Read the model definition and answer for the solid it produces. Units are mm, in the model's axes. A direction names the side the tool comes from. Coordinates: 2 decimals unless noted, no trailing zeros. Loops run counter-clockwise (first coordinate to the right, second up) from the corner with the lowest first, then second, coordinate; pieces in that order, holes last.
from build123d import *

# Parameters (mm, degrees)
SKETCH021_W       = 18.9
SKETCH021_H       = 58
EXTRUDE021_DEPTH  = 10
SKETCH020_W       = 90
SKETCH020_H       = 50
EXTRUDE020_DEPTH  = 200
CYLINDER_R        = 2.5
CYLINDER_DEPTH    = 70
CYLINDER002_R     = 2.5
CYLINDER002_DEPTH = 70
BOX001_W          = 82
BOX001_H          = 58
BOX001_DEPTH      = 44.4
BOX011_W          = 5
BOX011_H          = 5
BOX011_DEPTH      = 44.4
SKETCH001_R       = 5
EXTRUDE001_DEPTH  = 4
EXTRUDE002_DEPTH  = 15
SKETCH010_R       = 12.3
EXTRUDE010_DEPTH  = 5
BOX_W             = 75.7
BOX_H             = 45
BOX_DEPTH         = 44.4
BOX008_W          = 68.15
BOX008_H          = 15
BOX008_DEPTH      = 50
BOX009_W          = 68.15
BOX009_H          = 15
BOX009_DEPTH      = 50
BOX012_W          = 30
BOX012_H          = 100
BOX012_DEPTH      = 70
EXTRUDE003_DEPTH  = 25
BOX010_W          = 40
BOX010_H          = 120
BOX010_DEPTH      = 60
TUBE_R            = 45
TUBE_R_2          = 19.07
TUBE_DEPTH        = 50
BOX002_W          = 175
BOX002_H          = 90
BOX002_DEPTH      = 50
SKETCH016_W       = 10
SKETCH016_H       = 33.333334
EXTRUDE016_DEPTH  = 80
SKETCH_W          = 20
SKETCH_H          = 100
EXTRUDE_DEPTH     = 100
BOX017_W          = 120
BOX017_H          = 100
BOX017_DEPTH      = 70


with BuildPart() as extrude021:
    # Sketch021 (on Face14 of Cut017) → Extrude021 (new body)
    with BuildSketch(Plane(origin=(0, 0, 44.4), x_dir=(1, 0, 0), z_dir=(0, 0, -1))):
        with Locations((-72.55, -19.37)):
            Rectangle(SKETCH021_W, SKETCH021_H)
    extrude(amount=-EXTRUDE021_DEPTH)


with BuildPart() as extrude020:
    # Sketch020 (on Face26 of Cut016) → Extrude020 (new body)
    with BuildSketch(Plane.YZ.offset(-92)):
        with Locations((19, 15)):
            Rectangle(SKETCH020_W, SKETCH020_H)
    extrude(amount=EXTRUDE020_DEPTH)


with BuildPart() as throughholecylinder2:
    # Cylinder → Cylinder (new body)
    with BuildSketch(Plane(origin=(-86, -18, -20), x_dir=(1, 0, 0), z_dir=(0, 0, 1))):
        Circle(CYLINDER_R)
    extrude(amount=CYLINDER_DEPTH)


with BuildPart() as throughholecylinder1:
    # Cylinder002 → Cylinder002 (new body)
    with BuildSketch(Plane(origin=(-86, 56, -20), x_dir=(1, 0, 0), z_dir=(0, 0, 1))):
        Circle(CYLINDER002_R)
    extrude(amount=CYLINDER002_DEPTH)


with BuildPart() as motorhead:
    # Box001 → Box001 (new body)
    with BuildSketch(Plane(origin=(-82, -9.63, 0), x_dir=(1, 0, 0), z_dir=(0, 0, 1))):
        with Locations((41, 29)):
            Rectangle(BOX001_W, BOX001_H)
    extrude(amount=BOX001_DEPTH)


with BuildPart() as obj1:
    # Box011 → Box011 (new body)
    with BuildSketch(Plane(origin=(75.7, 16.87, 0), x_dir=(1, 0, 0), z_dir=(0, 0, 1))):
        with Locations((2.5, 2.5)):
            Rectangle(BOX011_W, BOX011_H)
    extrude(amount=BOX011_DEPTH)


with BuildPart() as obj2:
    # Sketch001 (on Face3 of Extrude010) → Extrude001 (new body)
    with BuildSketch(Plane.XY.offset(49.4)):
        with Locations((-58.7, 20.37)):
            Circle(SKETCH001_R)
    extrude(amount=EXTRUDE001_DEPTH)


with BuildPart() as obj3:
    # Sketch002 (on Face3 of Extrude001) → Extrude002 (new body)
    with BuildSketch(Plane.XY.offset(53.4)):
        with BuildLine():
            Line((-62.7, 23.37), (-62.7, 17.37))
            ThreePointArc((-62.7, 17.37), (-53.7, 20.37), (-62.7, 23.37))
        make_face()
    extrude(amount=EXTRUDE002_DEPTH)


with BuildPart() as motorshaftassembly:
    # Sketch010 (on Face6 of Box001) → Extrude010 (new body)
    with BuildSketch(Plane(origin=(-82, -9.63, 44.4), x_dir=(1, 0, 0), z_dir=(0, 0, 1))):
        with Locations((23.3, 30)):
            Circle(SKETCH010_R)
    extrude(amount=EXTRUDE010_DEPTH)

    # Fusion002: union obj2, obj3
    add(obj2.part)
    add(obj3.part)


with BuildPart() as motor:
    # Box → Box (new body)
    with BuildSketch(Plane(origin=(0, -3.13, 0), x_dir=(1, 0, 0), z_dir=(0, 0, 1))):
        with Locations((37.85, 22.5)):
            Rectangle(BOX_W, BOX_H)
    extrude(amount=BOX_DEPTH)

    # Fusion005: union MotorHead, obj1, MotorShaftAssembly
    add(motorhead.part)
    add(obj1.part)
    add(motorshaftassembly.part)


with BuildPart() as cube008:
    # Box008 → Box008 (new body)
    with BuildSketch(Plane(origin=(41, -26, -10), x_dir=(1, 0, 0), z_dir=(0, 0, 1))):
        with Locations((34.075, 7.5)):
            Rectangle(BOX008_W, BOX008_H)
    extrude(amount=BOX008_DEPTH)


with BuildPart() as cube009:
    # Box009 → Box009 (new body)
    with BuildSketch(Plane(origin=(41, 49, -10), x_dir=(1, 0, 0), z_dir=(0, 0, 1))):
        with Locations((34.075, 7.5)):
            Rectangle(BOX009_W, BOX009_H)
    extrude(amount=BOX009_DEPTH)


with BuildPart() as steeringshaftcutter:
    # Box012 → Box012 (new body)
    with BuildSketch(Plane(origin=(136, -31, -14), x_dir=(1, 0, 0), z_dir=(0, 0, 1))):
        with Locations((15, 50)):
            Rectangle(BOX012_W, BOX012_H)
    extrude(amount=BOX012_DEPTH)


with BuildPart() as fingers:
    # Sketch004 (on Face2 of Tube) → Extrude003 (new body)
    with BuildSketch(Plane(origin=(120.15, 19, 40), x_dir=(1, 0, 0), z_dir=(0, 0, 1))):
        with BuildLine():
            Line((16.519435, -9.5375), (20.849562, -12.0375))
            ThreePointArc((12.0375, -20.849562), (17.023596, -17.023596), (20.849562, -12.0375))
            Line((12.0375, -20.849562), (9.5375, -16.519435))
            ThreePointArc((9.5375, -16.519435), (13.488062, -13.488062), (16.519435, -9.5375))
        make_face()
        with BuildLine():
            Line((0, -24.075), (0, -19.07))
            ThreePointArc((-9.535, -16.515104), (-4.935679, -18.420206), (0, -19.07))
            Line((-9.535, -16.515104), (-12.0375, -20.849562))
            ThreePointArc((-12.0375, -20.849562), (-6.231069, -23.254664), (0, -24.075))
        make_face()
        with BuildLine():
            Line((-20.849562, -12.0375), (-16.515104, -9.535))
            ThreePointArc((-19.07, 0), (-18.420206, -4.935679), (-16.515104, -9.535))
            Line((-19.07, 0), (-24.075, 0))
            ThreePointArc((-24.075, 0), (-23.254664, -6.231069), (-20.849562, -12.0375))
        make_face()
        with BuildLine():
            Line((-16.519435, 9.5375), (-20.849562, 12.0375))
            ThreePointArc((-12.0375, 20.849562), (-17.023596, 17.023596), (-20.849562, 12.0375))
            Line((-12.0375, 20.849562), (-9.5375, 16.519435))
            ThreePointArc((-9.5375, 16.519435), (-13.488062, 13.488062), (-16.519435, 9.5375))
        make_face()
        with BuildLine():
            Line((0, 24.075), (0, 19.075))
            ThreePointArc((9.5375, 16.519435), (4.936973, 18.425035), (0, 19.075))
            Line((9.5375, 16.519435), (12.0375, 20.849562))
            ThreePointArc((12.0375, 20.849562), (6.231069, 23.254664), (0, 24.075))
        make_face()
        with BuildLine():
            Line((16.515104, 9.535), (20.849562, 12.0375))
            ThreePointArc((24.075, 0), (23.254664, 6.231069), (20.849562, 12.0375))
            Line((19.07, 0), (24.075, 0))
            ThreePointArc((19.07, 0), (18.420206, 4.935679), (16.515104, 9.535))
        make_face()
    extrude(amount=EXTRUDE003_DEPTH)


with BuildPart() as fingers_1:
    # Extrude003 placement: moved
    add(fingers.part.moved(Location((0, 0, -5))))


with BuildPart() as obj4:
    # Box010 → Box010 (new body)
    with BuildSketch(Plane(origin=(55, -34, -17), x_dir=(1, 0, 0), z_dir=(0, 0, 1))):
        with Locations((20, 60)):
            Rectangle(BOX010_W, BOX010_H)
    extrude(amount=BOX010_DEPTH)


with BuildPart() as steeringshaftcutdown:
    # Tube → Tube (new body)
    with BuildSketch(Plane(origin=(120.15, 19, -10), x_dir=(1, 0, 0), z_dir=(0, 0, 1))):
        Circle(TUBE_R)
        Circle(TUBE_R_2, mode=Mode.SUBTRACT)
    extrude(amount=TUBE_DEPTH)

    # Cut005: cut obj4
    add(obj4.part, mode=Mode.SUBTRACT)

    # Fusion004: union Fingers
    add(fingers_1.part)


with BuildPart() as steeringshaftcutdown_1:
    # Fusion004 placement: moved
    add(steeringshaftcutdown.part.moved(Location((-12, 0, 0))))

    # Cut006: cut SteeringShaftCutter
    add(steeringshaftcutter.part, mode=Mode.SUBTRACT)


with BuildPart() as motormount:
    # Box002 → Box002 (new body)
    with BuildSketch(Plane(origin=(-92, -26, -10), x_dir=(1, 0, 0), z_dir=(0, 0, 1))):
        with Locations((87.5, 45)):
            Rectangle(BOX002_W, BOX002_H)
    extrude(amount=BOX002_DEPTH)

    # Fusion: union Motor, Cube008, Cube009, SteeringShaftCutDown
    add(motor.part)
    add(cube008.part)
    add(cube009.part)
    add(steeringshaftcutdown_1.part)

    # Cut: cut ThroughHoleCylinder1
    add(throughholecylinder1.part, mode=Mode.SUBTRACT)

    # Cut013: cut ThroughHoleCylinder2
    add(throughholecylinder2.part, mode=Mode.SUBTRACT)


with BuildPart() as extrude016:
    # Sketch016 (on Face6 of Extrude) → Extrude016 (new body)
    with BuildSketch(Plane.XY.offset(150)):
        with Locations((-168.1, 18.7)):
            Rectangle(SKETCH016_W, SKETCH016_H)
    extrude(amount=-EXTRUDE016_DEPTH)


with BuildPart() as cut015:
    # Sketch (on Face6 of Box017) → Extrude (new body)
    with BuildSketch(Plane(origin=(-183.1, -31.3, 50), x_dir=(1, 0, 0), z_dir=(0, 0, 1))):
        with Locations((10, 50)):
            Rectangle(SKETCH_W, SKETCH_H)
    extrude(amount=EXTRUDE_DEPTH)

    # Cut015: cut Extrude016
    add(extrude016.part, mode=Mode.SUBTRACT)


with BuildPart() as cut018:
    # Box017 → Box017 (new body)
    with BuildSketch(Plane(origin=(-183.1, -31.3, -20), x_dir=(1, 0, 0), z_dir=(0, 0, 1))):
        with Locations((60, 50)):
            Rectangle(BOX017_W, BOX017_H)
    extrude(amount=BOX017_DEPTH)

    # Fusion013: union Cut015
    add(cut015.part)

    # Cut016: cut MotorMount
    add(motormount.part, mode=Mode.SUBTRACT)

    # Cut017: cut Extrude020
    add(extrude020.part, mode=Mode.SUBTRACT)

    # Cut018: cut Extrude021
    add(extrude021.part, mode=Mode.SUBTRACT)


solid = cut018.part
Q1. Flat-ended cylindrical pins translate along their axes: pin 1 Ø8.5 at (x, y) = (-77, 14.5) entering from +Z; pin 2 Ø8 at (x, y) = (-99.5, 0) entering from +Z; pin 3 Ø16.5 at (y, z) = (20, 108) entering from +X. Find the tip coordinate at first contact, or state that the pin passes through.
Findings below:
pin 1: stops at z = -10
pin 2: stops at z = 50
pin 3: stops at x = -173.1
Q2. A cutting plane is placed at A-A (x = -166). Give the vertices of the cut face in (y, z), then the cut area to 3 significant figures.
Findings below:
outline: (-31.3, -20) - (68.7, -20) - (68.7, 150) - (35.37, 150) - (35.37, 70) - (2.03, 70) - (2.03, 150) - (-31.3, 150) - close
area: 14,300 mm2
Q3. A cutting plane is placed at D-D (y = -16.5). Give the vertices of the cut face in (x, z), then the cut area to 4 significant figures.
Findings below:
outline: (-183.1, -20) - (-63.1, -20) - (-63.1, -10) - (-92, -10) - (-92, 40) - (-63.1, 40) - (-63.1, 50) - (-163.1, 50) - (-163.1, 150) - (-183.1, 150) - close
area: 8,955 mm2
Q4. A cutting plane is placed at B-B (y = 25). Give the vertices of the cut face in (x, z).
Findings below:
outline: (-183.1, -20) - (-63.1, -20) - (-63.1, -10) - (-92, -10) - (-92, 40) - (-82, 40) - (-82, 50) - (-163.1, 50) - (-163.1, 70) - (-173.1, 70) - (-173.1, 150) - (-183.1, 150) - close
Q5. A cutting plane is placed at C-C (z = 35). Give the vertices of the cut face in (x, y).
Findings below:
outline: (-183.1, -31.3) - (-63.1, -31.3) - (-63.1, -26) - (-92, -26) - (-92, 64) - (-63.1, 64) - (-63.1, 68.7) - (-183.1, 68.7) - close
Q6. Determine the mould class of faces 1 (the face through (-183.1, 18, 64)), 2 (the face through (-168, 19, 70)), 3 (the face through (-137, -31.3, 26)), 4 (the face through (-78, -26, 15)) for opening direction Y: +Y half, -Y half, draft (parallel to the pull), parting line (faces both ways), or undercut.
Findings below:
face 1: draft
face 2: undercut
face 3: -Y half
face 4: undercut
Q7. Which of the six approach directions +Z, -Z, +X, -X, +Y, -Y give full straight-line access (tool end or side, diameter ignored) to faces 5 (the face through (-78, 20, -10)), 6 (the face through (-82, 20, 45)), 7 (the face through (-175, 19, 150)), 8 (the face through (-163.1, 40, 99)), 9 (the face through (-137, 68.7, 26))?
Findings below:
face 5: +X
face 6: +Z, +X
face 7: +Z, +X, -X, +Y, -Y
face 8: +Z, +X, +Y, -Y
face 9: +Z, -Z, +X, -X, +Y
Q8. Straight lines are drawn through the part: probe 1 along X at (y, z) = (59.5, 81.5); probe 2 along Z at (x, y) = (-90, 55.5); probe 3 along X at (y, z) = (1, -2). For each, find the intervals that lie inside material, in ascending order.
Findings below:
probe 1: x = -183.1 to -163.1
probe 2: z = -20 to -10, 40 to 50
probe 3: x = -183.1 to -92
